```python
from build123d import *

# Parameters (mm, degrees)
F0_W     = 98
F0_H     = 25
F0_R     = 6
F1_DEPTH = 25
F3_START = 35
F2_R     = 3.4
F3_DEPTH = 85
F7_START = -35
F6_R     = 8
F7_DEPTH = 65
F8_SIZE  = 0.5
F9_SIZE  = 1


with BuildPart() as f1:
    # F0 (on Top) → F1 (new body)
    with BuildSketch(Plane.XY):
        Rectangle(F0_W, F0_H)
        with Locations((-20, 0)):
            Circle(F0_R, mode=Mode.SUBTRACT)
        with Locations((2, 0)):
            Circle(F0_R, mode=Mode.SUBTRACT)
        with Locations((24, 0)):
            Circle(F0_R, mode=Mode.SUBTRACT)
    extrude(amount=F1_DEPTH)

    # F2 (on Right) → F3 (cut)
    with BuildSketch(Plane.YZ.offset(F3_START)):
        with Locations((0, 12.5)):
            Circle(F2_R)
    extrude(amount=F3_DEPTH, mode=Mode.SUBTRACT)

    # F6 (on Right) → F7 (cut)
    with BuildSketch(Plane.YZ.offset(F7_START)):
        with Locations((0, 12.5)):
            Circle(F6_R)
    extrude(amount=-F7_DEPTH, mode=Mode.SUBTRACT)

    # F8
    f8_edges = [f1.edges().sort_by_distance(p)[0] for p in [
        (49, 12.5, 12.5),
        (49, -12.5, 12.5),
        (49, 0, 0),
        (49, 0, 25),
        (-49, 0, 25),
        (0, 12.5, 25),
        (0, -12.5, 25),
        (0, -12.5, 0),
        (-49, -12.5, 12.5),
        (-49, 0, 0),
        (-49, 12.5, 12.5),
        (0, 12.5, 0),
    ]]
    chamfer(f8_edges, length=F8_SIZE)

    # F9
    f9_edges = [f1.edges().sort_by_distance(p)[0] for p in [
        (-4, 0, 0),
        (18, 0, 0),
        (-26, 0, 0),
        (-26, 0, 25),
        (-4, 0, 25),
        (18, 0, 25),
    ]]
    chamfer(f9_edges, length=F9_SIZE)


solid = f1.part
```
CAD build for the part. Positions are in the model's coordinates, mm. A direction names the side the tool comes from. Round coordinates to 2 decimals unless told otherwise and drop trailing zeros. Write each loop counter-clockwise with the first axis right and the second up, starting at its lowest first coordinate (ties: lowest second). Pieces come first, ordered by that corner, then holes. Notation, with made-up numbers: (36, 54.5) -> (64, 54.5) arc R13 ccw to (64, 60.5) -> close; hole circle Ø5 at (11, 68.5). An arc over 180 degrees is marked (long way). Answer in a Markdown table with one row per item. Add a question column.
Item 1: Mould opens along Y. For faces 3 (the face through (35, 0, 13)), 4 (the face through (-1, -12.5, 12)), 5 (the face through (41.9, -0.74, 9.18)), 6 (the face through (-1, 8, 25)) say: pulls with the +Y half, pulls with the -Y half, needs draft (parallel to the pull), parting line crosses it, or undercut.
Item 2: Saw through at B-B, the plane x = 24. Write the cut outline in (y, z).
Item 3: Which spindle directions (+Z, -Z, +X, -X, +Y, -Y) get a long thin tool onto all of the face, cutting with end or side? Do faces 1 (the face through (19.24, -3.65, 12.34)), 2 (the face through (-41.9, -1.73, 4.69)). Say none if no direction does.
Item 4: Drop flat-ended pins along their axis: pin 1 Ø3 at (y, z) = (-2, 13.5) entering from -X; pin 2 Ø4 at (y, z) = (0, 12.5) entering from +X; pin 3 Ø1.5 at (x, y) = (-9.5, -5.5) entering from -Z. Give the stop position or say it passes through.
Item 5: Saw through at A-A, the plane z = 3. Write the cut outline in (x, y).
Item 6: Saw through at C-C, the plane x = -41. Write the cut outline in (y, z), then the cut area to 3 significant figures.
Item 7: Drill centre lines: line 1 (X direction, y = 5, z = 22); line 2 (X direction, y = -5.5, z = 14.5); line 3 (Y direction, x = 2, z = 11). Where is each one in solid material? Low to high. Write a range as from..to.
Item 8: Saw through at D-D, the plane y = 0. Count the separate pieces of the cut face and the enclosed holes in it, then the cut area to 3 significant figures.
Findings below:
| question | item | result |
|---|---|---|
| 1 | face 3 | undercut |
| 1 | face 4 | pulls with the -Y half |
| 1 | face 5 | undercut |
| 1 | face 6 | needs draft |
| 2 | outline | (-12.5, 0.5) -> (-12, 0) -> (-7, 0) -> (-6, 1) -> (-6, 24) -> (-7, 25) -> (-12, 25) -> (-12.5, 24.5) -> close; (6, 1) -> (7, 0) -> (12, 0) -> (12.5, 0.5) -> (12.5, 24.5) -> (12, 25) -> (7, 25) -> (6, 24) -> close |
| 3 | face 1 | +Z, -Z |
| 3 | face 2 | -X |
| 4 | pin 1 | stops at x = -35 |
| 4 | pin 2 | stops at x = 35 |
| 4 | pin 3 | stops at z = 0 |
| 5 | outline | (-49, -12) -> (-48.5, -12.5) -> (48.5, -12.5) -> (49, -12) -> (49, 12) -> (48.5, 12.5) -> (-48.5, 12.5) -> (-49, 12) -> close; hole circle Ø12 at (-20, 0); hole circle Ø12 at (2, 0); hole circle Ø12 at (24, 0) |
| 6 | outline | (-12.5, 0.5) -> (-12, 0) -> (12, 0) -> (12.5, 0.5) -> (12.5, 24.5) -> (12, 25) -> (-12, 25) -> (-12.5, 24.5) -> close; hole circle Ø16 at (0, 12.5) |
| 6 | area | 423 mm^2 |
| 7 | line 1 | x = -49..-23.32, -16.68..-1.32, 5.32..20.68, 27.32..49 |
| 7 | line 2 | x = -35..-22.4, -17.6..-0.4, 4.4..21.6, 26.4..49 |
| 7 | line 3 | y = -12.5..-6, 6..12.5 |
| 8 | separate pieces | 4 |
| 8 | enclosed holes | 0 |
| 8 | area | 1,220 mm^2 |
